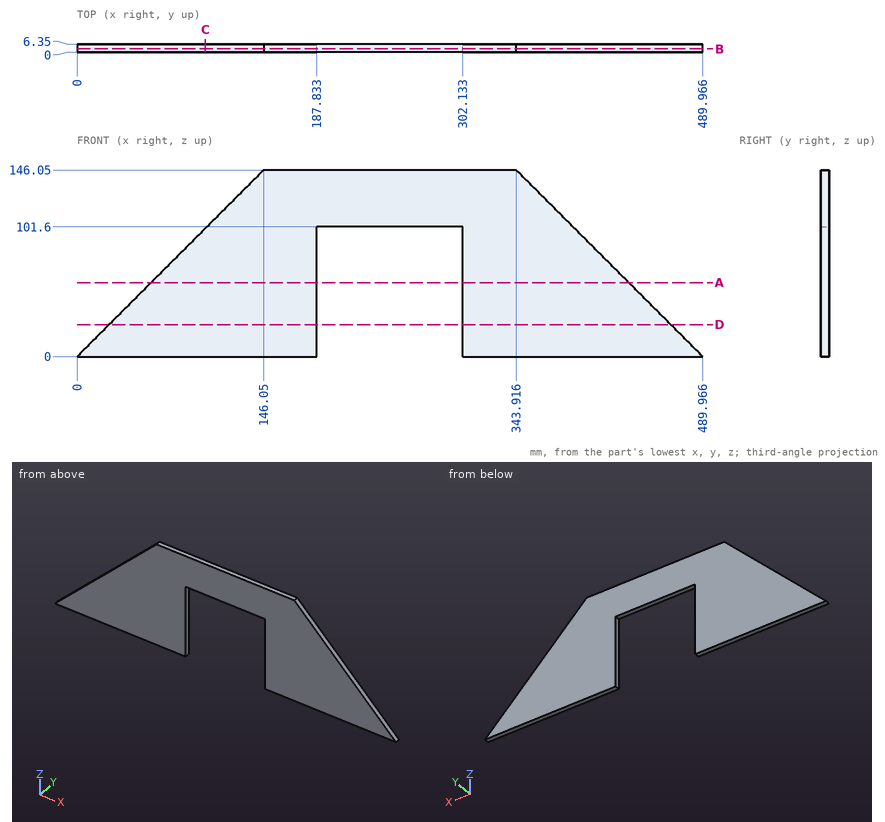
Answer from the drawing. Dimensions are ordinates in mm from the lowest x, y and z of the part. Give positions to 0.01 mm unless a question says otherwise; leave off trailing zeros. Loops run counter-clockwise (first coordinate to the right, second up) from the corner with the lowest first, then second, coordinate; pieces in that order, holes last. Notation, with made-up numbers: (-28, 37) - (25, 37) arc R21 ccw to (25, 76) - close; hole circle Ø9 at (73.25, -27). An arc over 180 degrees is marked (long way). Write each question's results on one line, items separated by ' | '.
1. Find section A-A, the plane z = 58. Write down the section's boundary in (x, y).
Resolved:
outline: (58, 0) - (187.83, 0) - (187.83, 6.35) - (58, 6.35) - close; (302.13, 0) - (431.97, 0) - (431.97, 6.35) - (302.13, 6.35) - close
2. Flat-ended cylindrical pins translate along their axes: P1, Ø1, axis at x = 358, y = 3, coming from the +Z side; P2, Ø1, axis at y = 4, z = 111.5, coming from the -X side; P3, Ø1.9, axis at x = 268, y = 2.5, coming from the -Z side; P4, Ø2, axis at x = 138, y = 5.5, coming from the -Z side. Find the tip coordinate at first contact, or state that the pin passes through.
Resolved:
P1: stops at z = 132.47 | P2: stops at x = 111 | P3: stops at z = 101.6 | P4: stops at z = 0
3. Find section D-D, the plane z = 25. Write down the section's boundary in (x, y).
Resolved:
outline: (25, 0) - (187.83, 0) - (187.83, 6.35) - (25, 6.35) - close; (302.13, 0) - (464.97, 0) - (464.97, 6.35) - (302.13, 6.35) - close
4. Consider probe 1 along Z at (x, y) = (219, 4.25); probe 2 along X at (y, z) = (2.25, 28.5); probe 3 along X at (y, z) = (1, 38). Determine where each line is inside the solid, lowest interval first. Write a range as from..to.
Resolved:
probe 1: z = 101.6..146.05 | probe 2: x = 28.5..187.83, 302.13..461.47 | probe 3: x = 38..187.83, 302.13..451.97
5. Find section C-C, the plane x = 100.5. Write down the section's boundary in (y, z), then the cut area to 3 significant figures.
Resolved:
outline: (0, 0) - (6.35, 0) - (6.35, 100.5) - (0, 100.5) - close | area: 638 mm^2
6. Find section B-B, the plane y = 2.5. Write down the section's boundary in (x, z), then the cut area to 3 significant figures.
Resolved:
outline: (0, 0) - (187.83, 0) - (187.83, 101.6) - (302.13, 101.6) - (302.13, 0) - (489.97, 0) - (343.92, 146.05) - (146.05, 146.05) - close | area: 38,600 mm^2
